Build history of the part. All positions in model axes, mm. A direction names the side the tool comes from. Give positions to 0.01 mm unless a question says otherwise; leave off trailing zeros. Loops run counter-clockwise (first coordinate to the right, second up) from the corner with the lowest first, then second, coordinate; pieces in that order, holes last.
1) Wall check: line 1 (Z direction, x = 25.5, y = 0); line 2 (Z direction, x = 7, y = 0); line 3 (X direction, y = -92, z = 25.5). Give the ranges that are in metal, low to high.
2) Flat gauge pins, fed straight in: P1, Ø1, axis at x = 23.5, z = 63.5, coming from the -Y side; P2, Ø10, axis at x = 28.5, z = -77.5, coming from the -Y side; P3, Ø8, axis at x = 33, z = -94.5, coming from the +Y side; P4, Ø5, axis at y = 49, z = -27.5, coming from the -X side. Where does each tip first touch, or does it go through?
3) Two-plate mould, pull along Y, no slides. Class faces 1 (the cylindrical face through (33.944, -7.509, -23.846)), 2 (the flat face through (10, 6, -5)), 3 (the cylindrical face through (23.804, 7.484, 0.494)), 4 (the flat face through (38, 6, -5)): +Y half, -Y half, draft (parallel to the pull), parting line (faces both ways), or undercut.
4) Band-saw the part on A-A on z = 0. List the corners of the cut face in (x, y), then the cut area to 3 significant figures.
5) Band-saw the part on C-C on x = 5. List the corners of the cut face in (y, z).
6) Band-saw the part on D-D on z = -87.5. List the corners of the cut face in (x, y), then the cut area to 3 significant figures.
7) 3-axis set-ups, long thin cutter, end or side, ignore diameter. For faces 5 (the cylindrical face through (14.79, -119.884, -5.276)), 6 (the cylindrical face through (4.93, 23.846, -7.509)), 7 (the flat face through (30, -2, 28)): which of +Z, -Z, +X, -X, +Y, -Y reach the whole face in a straight line?
Autodesk Inventor part; units mm, degrees
ref_plane "YZ Plane" through (0, 0, 0) normal (1, 0, 0) x (0, 1, 0)
ref_plane "XZ Plane" through (0, 0, 0) normal (0, 1, 0) x (-1, 0, 0)
ref_plane "XY Plane" through (0, 0, 0) normal (0, 0, 1) x (1, 0, 0)
sketch "Sketch1" plane through (0, 0, 0) normal (1, 0, 0) x (0, 1, 0)
  circle A0 centre (0, 0) radius 120
  circle A1 centre (0, 0) radius 25
  circle A2 centre (0, 0) radius 7.5
  dimension "d0" = 240
  dimension "d1" = 50
  dimension "d2" = 15
extrude "Extrusion1" add sketch "Sketch1" along normal blind 30 contours A0
sketch "Sketch2" plane through (30, 0, 0) normal (1, 0, 0) x (0, 0, -1)
  circle A0 centre (0, 0) radius 25
extrude "Extrusion2" add sketch "Sketch2" against normal blind 20
sketch "Sketch3" plane through (10, 0, 0) normal (-1, 0, 0) x (0, 0, 1)
  circle A0 centre (0, 0) radius 7.5
  dimension "d7" = 15
extrude "Extrusion3" cut sketch "Sketch3" against normal blind 20
sketch "Sketch4" plane through (30, 0, 0) normal (1, 0, 0) x (0, 0, -1)
  circle A0 centre (0, 0) radius 7.5
  circle A1 centre (0, 0) radius 25
  dimension "d10" = 50
extrude "Extrusion4" add sketch "Sketch4" along normal blind 8
properties part number "wheel"
Findings below:
1. line 1: z = -120 to -7.5, 7.5 to 120
1. line 2: z = -120 to -25, 25 to 120
1. line 3: x = 0 to 30
2. P1: stops at y = -102.13
2. P2: stops at y = -95.62
2. P3: stops at y = 77.22
2. P4: stops at x = 0
3. face 1: parting line
3. face 2: undercut
3. face 3: undercut
3. face 4: draft
4. outline: (0, -120) - (30, -120) - (30, -25) - (38, -25) - (38, -7.5) - (10, -7.5) - (10, -25) - (0, -25) - close; (0, 25) - (10, 25) - (10, 7.5) - (38, 7.5) - (38, 25) - (30, 25) - (30, 120) - (0, 120) - close
4. area: 6,680 mm2
5. outline: circle Ø240 at (0, 0); hole circle Ø50 at (0, 0)
6. outline: (0, -82.12) - (30, -82.12) - (30, 82.12) - (0, 82.12) - close
6. area: 4,930 mm2
7. face 5: +X, -X
7. face 6: -X
7. face 7: +X
